The drawing under review shows one solid part. Ordinate dimensions are in mm from its lowest x, y, z. Give positions to 0.01 mm unless a question says otherwise; leave off trailing zeros. Loops run counter-clockwise (first coordinate to the right, second up) from the corner with the lowest first, then second, coordinate; pieces in that order, holes last. Notation, with made-up numbers: M 50,41 L 85,41 A20 ccw 85,71 Z; hole C 82,50.25 d4. An arc over 180 degrees is marked long. Write item = value, one per line. Start each with the question number.
1. Wall thickness on line 1 along X through (y, z) = (23.25, 3.5); line 2 along X through (y, z) = (25, 2.75); line 3 along Z through (x, y) = (2.25, 28): over which ranges is each line inside the solid? List them lowest first. Write a range as from..to.
2. We need section C-C on y = 13.5. Give the boundary of the cut face in (x, z), then the cut area to 3 significant figures.
3. Draft analysis for pull direction X (two halves, no side actions). For the marked faces 1, 2 and 3, state which applies: pulls with the +X half, pulls with the -X half, needs draft (parallel to the pull), parting line crosses it, or undercut.
4. We need section B-B on z = 3.5. Give the boundary of the cut face in (x, y).
5. We need section D-D on z = 6. Give the boundary of the cut face in (x, y).
6. For pin 1 (3 mm diameter, centred on x = 4, z = 1, fed in from -Y); pin 2 (2 mm diameter, centred on y = 8.5, z = 5, fed in from +X); pin 3 (2 mm diameter, centred on x = 3, z = 4.5, fed in from +Y); pin 4 (1.5 mm diameter, centred on x = 1, y = 5, fed in from -Z), all flat-tipped, find the tip position at first contact; note any pin that passes through.
7. We need section A-A on x = 3.5. Give the boundary of the cut face in (y, z), then the cut area to 3 significant figures.
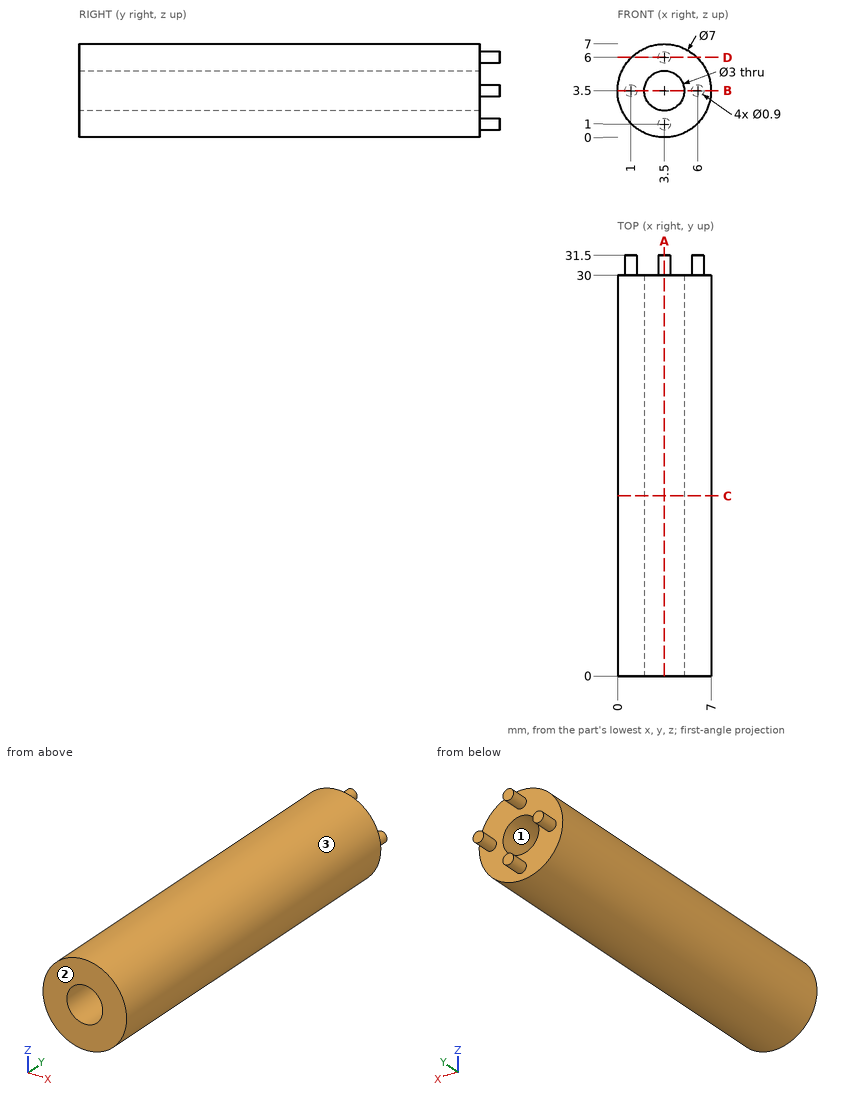
Final values:
q1.line_1 = 0..2, 5..7
q1.line_2 = 0.08..2.2, 4.8..6.92
q1.line_3 = 0.23..2.67, 4.33..6.77
q2.outline = C 3.5,3.5 d7; hole C 3.5,3.5 d3
q2.area = 31.4 mm²
q3.face_1 = undercut
q3.face_2 = needs draft
q3.face_3 = parting line crosses it
q4.outline = M 0,0 L 2,0 L 2,30 L 1.45,30 L 1.45,31.5 L 0.55,31.5 L 0.55,30 L 0,30 Z; M 5,0 L 7,0 L 7,30 L 6.45,30 L 6.45,31.5 L 5.55,31.5 L 5.55,30 L 5,30 Z
q5.outline = M 1.05,0 L 5.95,0 L 5.95,30 L 3.95,30 L 3.95,31.5 L 3.05,31.5 L 3.05,30 L 1.05,30 Z
q6.pin_1 = 0
q6.pin_2 = 6.96
q6.pin_3 = 30
q6.pin_4 = 0.47
q7.outline = M 0,0 L 30,0 L 30,0.55 L 31.5,0.55 L 31.5,1.45 L 30,1.45 L 30,2 L 0,2 Z; M 0,5 L 30,5 L 30,5.55 L 31.5,5.55 L 31.5,6.45 L 30,6.45 L 30,7 L 0,7 Z
q7.area = 123 mm²
